Part model, mm, in its own coordinate system. A direction names the side the tool comes from. Round coordinates to 2 decimals unless told otherwise and drop trailing zeros. Write each loop counter-clockwise with the first axis right and the second up, starting at its lowest first coordinate (ties: lowest second). Pieces come first, ordered by that corner, then holes. Notation, with made-up numbers: M 44.5,75.25 L 100.5,75.25 A20 cw 100.5,86.25 Z; hole C 48,75 d11. An arc over 180 degrees is marked long. Answer as a JSON object with one key per item and string values. Group by question number.
1. Band-saw the part on B-B, the plane z = 5. Write the cut outline in (x, y).
2. Band-saw the part on C-C, the plane z = 91. Write the cut outline in (x, y).
3. Band-saw the part on A-A, the plane y = 0. Write the cut outline in (x, z), plus the area to 3 significant figures.
4. Which spindle directions (+Z, -Z, +X, -X, +Y, -Y) get a long thin tool onto all of the face, cutting with end or side? Do faces 1 (the face through (2.769, -5.323, 52.265)), 2 (the face through (0, 4.5, 101)). Say none if no direction does.
5. Drill centre lines: line 1 (Z direction, x = 2.25, y = 0); line 2 (X direction, y = -4.5, z = 60.5); line 3 (Z direction, x = 5.5, y = 1). Where is each one in solid material? Low to high. Write a range as from..to.
6. Drop flat-ended pins along their axis: pin 1 (1 mm diameter, centred on x = 2.5, z = 90.5, fed in from +Y); pin 2 (0.5 mm diameter, centred on x = 0.5, y = 5.5, fed in from +Z); pin 3 (2.5 mm diameter, centred on y = 0, z = 5, fed in from -X). Give the stop position or say it passes through.
from build123d import *

# Parameters (mm, degrees)
SKETCH1_R               = 6
BOSS_EXTRUDE1_DEPTH     = 106
CHAMFER1_SIZE           = 0.5
SKETCH2_W               = 20
SKETCH2_H               = 5
CUT_EXTRUDE1_DEPTH      = 10
SKETCH3_R               = 1.5
CUT_EXTRUDE2_DEPTH      = 7
CUT_EXTRUDE2_DEPTH_BACK = 7


with BuildPart() as part:
    # Sketch1 → Boss-Extrude1 (new body)
    with BuildSketch(Plane.XY):
        Circle(SKETCH1_R)
    extrude(amount=BOSS_EXTRUDE1_DEPTH)

    # Chamfer1
    chamfer1_edges = [part.edges().sort_by_distance(p)[0] for p in [
        (-6, 0, 0),
        (-6, 0, 106),
    ]]
    chamfer(chamfer1_edges, length=CHAMFER1_SIZE)

    # Sketch2 → Cut-Extrude1 (cut)
    with BuildSketch(Plane.XY.offset(106)):
        with Locations((0, 7)):
            Rectangle(SKETCH2_W, SKETCH2_H)
    extrude(amount=-CUT_EXTRUDE1_DEPTH, mode=Mode.SUBTRACT)

    # Sketch3 → Cut-Extrude2 (cut, two sides)
    with BuildSketch(Plane(origin=(0, 0, 0), x_dir=(0, 0, -1), z_dir=(1, 0, 0))) as cut_extrude2_sk:
        with Locations((-5, 0)):
            Circle(SKETCH3_R)
    extrude(amount=CUT_EXTRUDE2_DEPTH, mode=Mode.SUBTRACT)
    extrude(cut_extrude2_sk.sketch, amount=-CUT_EXTRUDE2_DEPTH_BACK, mode=Mode.SUBTRACT)


solid = part.part
Worked answers:
{
 "1": {"outline": "M -5.81,-1.5 A6 ccw 5.81,-1.5 Z; M -5.81,1.5 L 5.81,1.5 A6 ccw Z"},
 "2": {"outline": "C 0,0 d12"},
 "3": {"outline": "M -6,0.5 L -5.5,0 L 5.5,0 L 6,0.5 L 6,3.5 L -6,3.5 Z; M -6,6.5 L 6,6.5 L 6,105.5 L 5.5,106 L -5.5,106 L -6,105.5 Z", "area": "1,240 mm^2"},
 "4": {"face 1": "+Z, -Z", "face 2": "+Z, +X, -X, +Y"},
 "5": {"line 1": "z = 0..3.5, 6.5..106", "line 2": "x = -3.97..3.97", "line 3": "z = 0.09..3.88, 6.12..105.91"},
 "6": {"pin 1": "stops at y = 5.66", "pin 2": "stops at z = 96", "pin 3": "passes through"}
}
